from build123d import *

# Parameters (mm, degrees)
SKETCH1_W            = 590.55
SKETCH1_H            = 114.3
BASE_FLANGE1_DEPTH   = 3.175
EDGE_FLANGE1_START   = -590.55
EDGE_FLANGE1_DEPTH   = 590.55
EDGE_FLANGE1_2_DEPTH = 590.55


# Read off the part's stored shape, not the designer's step: Edge-Flange1
# Sheet-metal steps are written as plain solids
with BuildPart() as part:
    # Sketch1 → Base-Flange1 (new body)
    with BuildSketch(Plane(origin=(0, 0, 0), x_dir=(0, 0, -1), z_dir=(1, 0, 0))):
        with Locations((295.275, 57.15)):
            Rectangle(SKETCH1_W, SKETCH1_H)
    extrude(amount=-BASE_FLANGE1_DEPTH)

    # Edge-Flange1 outline → Edge-Flange1 (cut)
    with BuildSketch(Plane.XY.offset(EDGE_FLANGE1_START)):
        with BuildLine():
            Line((-3.175, 114.3), (-3.175, 107.644005193))
            ThreePointArc((-3.175, 107.644005193), (-0.850738686, 105.319743879), (0, 102.144743879))
            Line((0, 102.144743879), (0, 114.3))
            Line((0, 114.3), (-3.175, 114.3))
        make_face()
    extrude(amount=EDGE_FLANGE1_DEPTH, mode=Mode.SUBTRACT)

    # Edge-Flange1 2 outline → Edge-Flange1 2 (add)
    with BuildSketch(Plane.XY.offset(EDGE_FLANGE1_START)):
        with BuildLine():
            ThreePointArc((-3.175, 107.644005193), (-7.178841321, 108.440418748), (-10.840128061, 106.634871939))
            Line((-10.840128061, 106.634871939), (-35.921024484, 81.553975516))
            Line((-35.921024484, 81.553975516), (-33.675960454, 79.308911485))
            Line((-33.675960454, 79.308911485), (-8.59506403, 104.389807909))
            ThreePointArc((-8.59506403, 104.389807909), (-5.134980102, 105.078061395), (-3.175, 102.144743879))
            Line((-3.175, 102.144743879), (-3.175, 107.644005193))
        make_face()
    extrude(amount=EDGE_FLANGE1_2_DEPTH)


solid = part.part
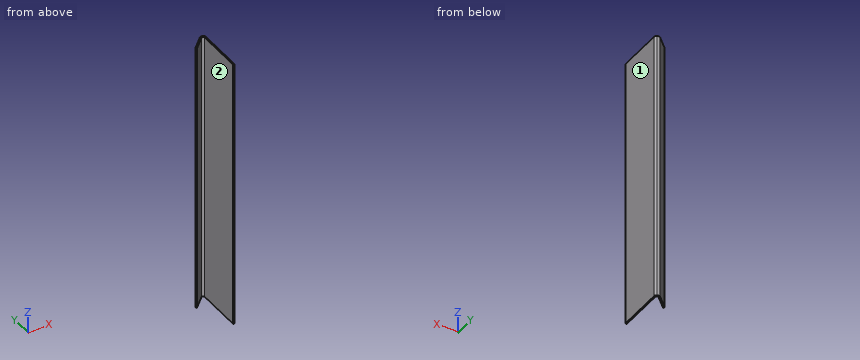
Read the model definition and answer for the solid it produces. Units are mm, in the model's axes. Face numbers are marked on the shaded views. Give positions to 0.01 mm unless a question says otherwise; leave off trailing zeros. Loops run counter-clockwise (first coordinate to the right, second up) from the corner with the lowest first, then second, coordinate; pieces in that order, holes last. Notation, with made-up numbers: (-19.75, 36) - (10.25, 36) arc R31 cw to (10.25, 64) - close; hole circle Ø8 at (42.5, -31.5). An arc over 180 degrees is marked (long way). Answer as CSV lines item,"result". Start each with the question number.
1) Straight lines are drawn through the part: L1, parallel to X at y = 28.5, z = -526 (3 decimals); L2, parallel to X at y = 94.5, z = -415 (3 decimals); L3, parallel to Y at x = -10.5, z = -147.5. For each, find the intervals that lie inside material, in ascending order. Write a range as from..to.
2) Find section C-C (y = 42.5). Write down the section's boundary in (x, z) (3 decimals), then the cut area to 4 significant figures.
3) Each of these flat-tipped pins is pushed along its axis until it touches: pin 1 Ø1.5 at (y, z) = (78.5, -396.5) entering from -X (3 decimals); pin 2 Ø1 at (x, z) = (-30, -379) entering from +Y (3 decimals). Where does it stop, or does it pass through?
4) Find section A-A (y = 95). Write down the section's boundary in (x, z) (3 decimals).
5) Find section D-D (x = -26.5). Write down the section's boundary in (y, z) (3 decimals).
6) Determine the mould class of the marked faces 1 and 2 for opening direction X: released by +X, released by -X, zero draft, split by the parting line, or undercut.
7) Find section B-B (z = -351). Write down the section's boundary in (x, y) (3 decimals).
Findings below:
1,L1,"-3.175..0"
1,L2,"-22.975..-18.485, -3.175..0"
1,L3,"102.48..106.95"
2,outline,"(-3.175, -590.55) - (0, -590.55) - (0, 0) - (-3.175, 0) - close"
2,area,"1,875 mm^2"
3,pin 1,"x = -3.175"
3,pin 2,"y = 87.975"
4,outline,"(-22.475, -590.55) - (-17.985, -590.55) - (-17.985, 0) - (-22.475, 0) - close; (-3.175, -590.55) - (0, -590.55) - (0, 0) - (-3.175, 0) - close"
5,outline,"(86.485, -590.55) - (90.975, -590.55) - (90.975, 0) - (86.485, 0) - close"
6,face 1,"released by +X"
6,face 2,"undercut"
7,outline,"(-35.921, 81.554) - (-33.676, 79.309) - (-8.595, 104.39) arc R3.175 cw to (-3.175, 102.145) - (-3.175, 0) - (0, 0) - (0, 102.145) arc R6.35 ccw to (-10.84, 106.635) - close"
